Geometry: see drawing. Coordinates: mm, zero at the bounding-box minimum. Round coordinates to 2 decimals unless told otherwise and drop trailing zeros. Write each loop counter-clockwise with the first axis right and the second up, starting at its lowest first coordinate (ties: lowest second). Pieces come first, ordered by that corner, then holes. Notation, with made-up numbers: (3.25, 46.5) -> (21.25, 46.5) arc R6 ccw to (21.25, 53.5) -> close; hole circle Ø6 at (-30, 16). An arc over 180 degrees is marked (long way). Write item = value, one per line.
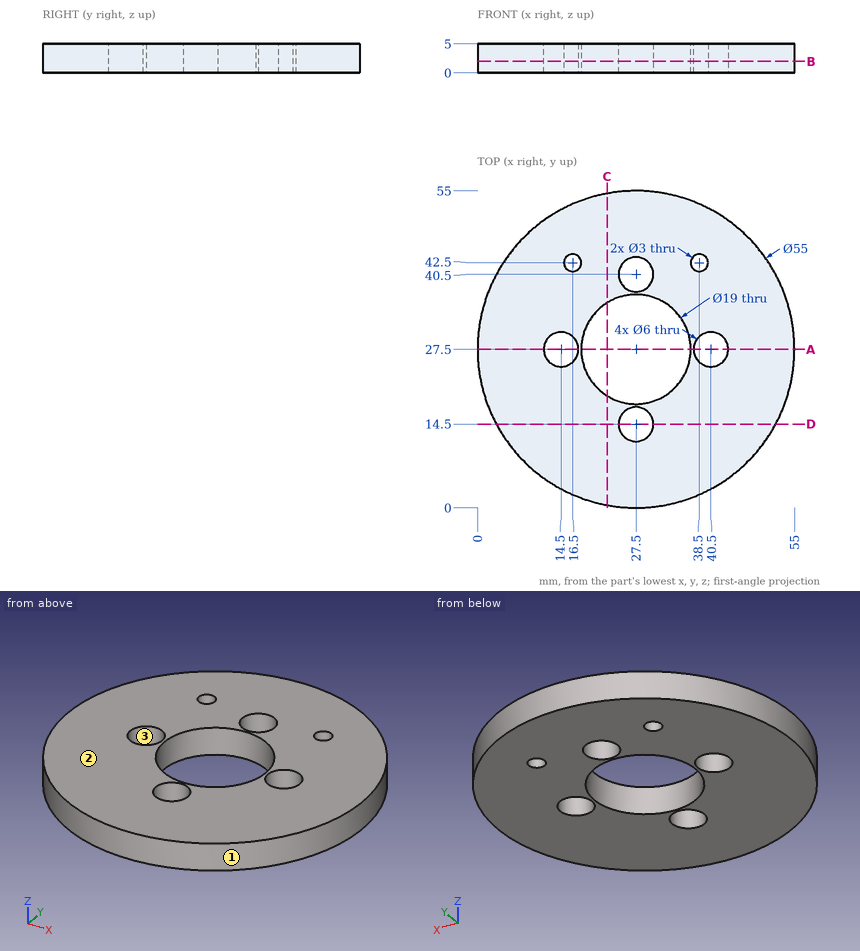
1) Cut plane A-A (y = 27.5). Return the cut outline in (x, z).
Solutions:
outline = (0, 0) -> (11.5, 0) -> (11.5, 5) -> (0, 5) -> close; (17.5, 0) -> (18, 0) -> (18, 5) -> (17.5, 5) -> close; (37, 0) -> (37.5, 0) -> (37.5, 5) -> (37, 5) -> close; (43.5, 0) -> (55, 0) -> (55, 5) -> (43.5, 5) -> close
2) Draft query along X for the marked faces 1, 2 and 3. Return one class per face: +X half, -X half, draft (parallel to the pull), parting line (faces both ways), or undercut.
Solutions:
face_1 = parting line
face_2 = draft
face_3 = undercut
3) First-contact query: P1, Ø1, axis at y = 49.5, z = 4, coming from the +X side. Flat tip, straight axial feed; report the tip coordinate or a pass-through.
Solutions:
P1 = 44.65
4) Cut plane C-C (x = 22.5). Return the cut outline in (y, z).
Solutions:
outline = (0.46, 0) -> (19.42, 0) -> (19.42, 5) -> (0.46, 5) -> close; (35.58, 0) -> (54.54, 0) -> (54.54, 5) -> (35.58, 5) -> close
5) Cut plane B-B (z = 2). Return the cut outline in (x, y), and give its area (3 significant figures).
Solutions:
outline = circle Ø55 at (27.5, 27.5); hole circle Ø6 at (14.5, 27.5); hole circle Ø3 at (16.5, 42.5); hole circle Ø19 at (27.5, 27.5); hole circle Ø6 at (27.5, 14.5); hole circle Ø6 at (27.5, 40.5); hole circle Ø3 at (38.5, 42.5); hole circle Ø6 at (40.5, 27.5)
area = 1,970 mm^2
6) Line query: L1, parallel to Y at x = 27.5, z = 1.25; L2, parallel to Y at x = 38.5, z = 2.8; L3, parallel to X at y = 15, z = 2.7. Output: solid intervals per line, ascending. Write a range as from..to.
Solutions:
L1 = 0..11.5, 17.5..18, 37..37.5, 43.5..55
L2 = 2.3..25.26, 29.74..41, 44..52.7
L3 = 3.01..24.54, 30.46..51.99
7) Cut plane D-D (y = 14.5). Return the cut outline in (x, z), and give its area (3 significant figures).
Solutions:
outline = (3.27, 0) -> (24.5, 0) -> (24.5, 5) -> (3.27, 5) -> close; (30.5, 0) -> (51.73, 0) -> (51.73, 5) -> (30.5, 5) -> close
area = 212 mm^2
